Check sheet for the modelled part. Datum: model origin and axes. Units: mm. A direction names the side the tool comes from. Round coordinates to 2 decimals unless told otherwise and drop trailing zeros. Write each loop counter-clockwise with the first axis right and the second up, starting at its lowest first coordinate (ties: lowest second). Pieces come first, ordered by that corner, then holes. Notation, with made-up numbers: (40.5, 12) -> (80.5, 12) arc R19 ccw to (80.5, 38) -> close; hole circle Ø7 at (33, 12). An arc over 180 degrees is marked (long way). One line per item, written item: value.
Autodesk Inventor part; units mm, degrees
ref_plane "YZ Plane" through (0, 0, 0) normal (1, 0, 0) x (0, 1, 0)
ref_plane "XZ Plane" through (0, 0, 0) normal (0, 1, 0) x (-1, 0, 0)
ref_plane "XY Plane" through (0, 0, 0) normal (0, 0, 1) x (1, 0, 0)
sketch "Sketch1" plane through (0, 0, 0) normal (0, 0, 1) x (1, 0, 0)
  circle A0 centre (0, 0) radius 46.5
extrude "Extrusion1" add sketch "Sketch1" along normal mid plane 6
sketch "Sketch2" plane through (0, 0, 3) normal (0, 0, 1) x (1, 0, 0)
  circle A0 centre (0, 0) radius 46.5
  circle A1 centre (0, 0) radius 4.5
  arc A2 (17.272, -47.4545) -> (50.5, 0) centre (0, 0) ccw
  line L0 (17.272, -47.4545) -> (4.2753, -11.7462)
  arc A3 (-6.25, -10.8253) -> (4.2753, -11.7462) centre (0, 0) ccw
  line L1 (-6.25, -10.8253) -> (-25.25, -43.7343)
  arc A4 (-49.7328, 8.7692) -> (-25.25, -43.7343) centre (0, 0) ccw
  line L2 (-49.7328, 8.7692) -> (-12.3101, 2.1706)
  arc A5 (-6.25, 10.8253) -> (-12.3101, 2.1706) centre (0, 0) ccw
  line L3 (-6.25, 10.8253) -> (-25.25, 43.7343)
  arc A6 (32.4608, 38.6852) -> (-25.25, 43.7343) centre (0, 0) ccw
  line L4 (32.4608, 38.6852) -> (8.0348, 9.5756)
  arc A7 (12.5, 0) -> (8.0348, 9.5756) centre (0, 0) ccw
  line L5 (12.5, 0) -> (50.5, 0)
  circle A8 centre (0, 0) radius 40.5 construction
  arc A9 (40.5, 0) -> (26.0329, 31.0248) centre (0, 0) ccw
  arc A10 (-20.25, 35.074) -> (-39.8847, 7.0328) centre (0, 0) ccw
  arc A11 (-20.25, -35.074) -> (13.8518, -38.0576) centre (0, 0) ccw
  point P0 (-23.25, -40.2702)
  point P1 (15.9039, -43.6957)
  point P2 (-23.25, 40.2702)
  point P3 (-45.7936, 8.0746)
  point P4 (46.5, 0)
  point P5 (29.8896, 35.6211)
  dimension "d4" = 6
extrude "Extrusion3" cut sketch "Sketch2" against normal through all contours L5 A7 L4 A9 | A11 L1 A3 L0 | L3 A5 L2 A10
sketch "Sketch3" plane through (0, 0, 3) normal (0, 0, 1) x (1, 0, 0)
  circle A0 centre (0, 0) radius 46.5
hole "Hole1" at (0, 0, 3) direction (0, 0, -1) diameter 8 end through all
properties part number "main_wheel"
Item 1: Sectioned sample at C-C on x = -29. Enter the section's corners in (y, z).
Answer:
outline: (-36.35, -3) -> (5.11, -3) -> (5.11, 3) -> (-36.35, 3) -> close; (28.27, -3) -> (36.35, -3) -> (36.35, 3) -> (28.27, 3) -> close
Item 2: Depth check by flat-ended pin: P1, Ø3, axis at x = -10.5, z = -1, coming from the -Y side; P2, Ø3, axis at x = 28.5, z = 2, coming from the +Y side; P3, Ø1, axis at y = -34, z = -1.5, coming from the +X side; P4, Ø6, axis at x = -6, y = -21, coming from the +Z side. Enter the tip coordinate at first touch or a pass-through.
Answer:
P1: stops at y = -45.62
P2: stops at y = 37.86
P3: stops at x = 32.25
P4: passes through
Item 3: Mould release check, pull along Y, two halves, no side actions. Record for faces 1 (the flat face through (-1, -10, -3)), 2 (the cylindrical face through (-10.195, 7.232, 0.042)), 3 (the cylindrical face through (44.35, 13.97, 0.04)): pulls with the +Y half, pulls with the -Y half, needs draft (parallel to the pull), parting line crosses it, or undercut.
Answer:
face 1: needs draft
face 2: undercut
face 3: parting line crosses it
Item 4: Tool access check on faces 4 (the flat face through (-1, -10, 3)), 5 (the cylindrical face through (11.361, 5.213, 0.042)). Record the directions out of +Z, -Z, +X, -X, +Y, -Y that give a thin tool (end or side, any length) a straight path to the whole face; none if there is none.
Answer:
face 4: +Z, +X, -X, +Y, -Y
face 5: +Z, -Z
Item 5: Sectioned sample at A-A on x = 0. Enter the section's corners in (y, z).
Answer:
outline: (-46.5, -3) -> (-40.5, -3) -> (-40.5, 3) -> (-46.5, 3) -> close; (-12.5, -3) -> (-4, -3) -> (-4, 3) -> (-12.5, 3) -> close; (4, -3) -> (46.5, -3) -> (46.5, 3) -> (4, 3) -> close
Item 6: Thickness scan on line 1 (Y direction, x = 0, z = -0.85); line 2 (Y direction, x = 1, z = -1.8); line 3 (X direction, y = 26.5, z = -1.35). Record the ranges inside material, lowest first.
Answer:
line 1: y = -46.5 to -40.5, -12.5 to -4, 4 to 46.5
line 2: y = -46.49 to -40.49, -12.46 to -3.87, 3.87 to 46.49
line 3: x = -38.21 to -30.63, -15.3 to 22.24, 30.63 to 38.21
Item 7: Sectioned sample at B-B on y = 33. Enter the section's corners in (x, z).
Answer:
outline: (-32.76, -3) -> (-23.48, -3) -> (-23.48, 3) -> (-32.76, 3) -> close; (-19.05, -3) -> (32.76, -3) -> (32.76, 3) -> (-19.05, 3) -> close
Item 8: Sectioned sample at D-D on z = -1.45. Enter the section's corners in (x, y).
Answer:
outline: circle Ø93 at (0, 0); hole (-39.88, 7.03) -> (-12.31, 2.17) arc R12.5 cw to (-6.25, 10.83) -> (-20.25, 35.07) arc R40.5 ccw to start; hole (-20.25, -35.07) arc R40.5 ccw to (13.85, -38.06) -> (4.28, -11.75) arc R12.5 cw to (-6.25, -10.83) -> close; hole circle Ø8 at (0, 0); hole (8.03, 9.58) arc R12.5 cw to (12.5, 0) -> (40.5, 0) arc R40.5 ccw to (26.03, 31.02) -> close
